Part model, mm, in its own coordinate system. Face numbers are marked on the shaded views. A direction names the side the tool comes from. Give positions to 0.01 mm unless a question says otherwise; leave off trailing zeros. Loops run counter-clockwise (first coordinate to the right, second up) from the corner with the lowest first, then second, coordinate; pieces in that order, holes last. Notation, with made-up numbers: M 33.5,-31 L 75.5,-31 A28 cw 75.5,-13 Z; hole C 43.5,27.5 d8. An arc over 180 degrees is marked long. Answer in a Markdown table with one row per item.
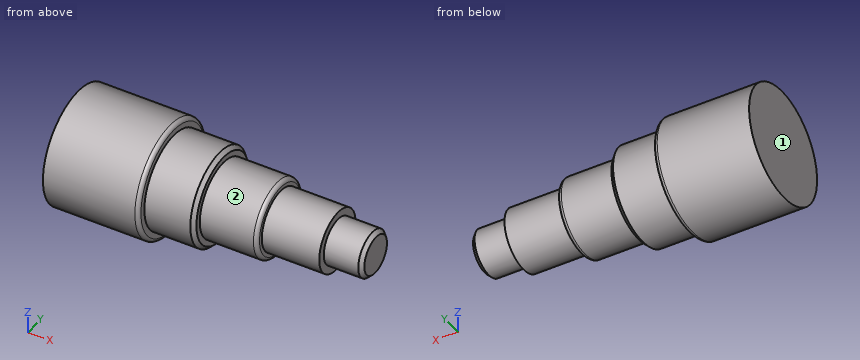
from build123d import *

# Parameters (mm, degrees)
F0_R     = 15
F1_DEPTH = 25
F2_R     = 12.5
F3_DEPTH = 13
F4_R     = 10
F5_DEPTH = 15
F6_R     = 8
F7_DEPTH = 15
F8_R     = 6
F9_DEPTH = 10
F10_R    = 1
F11_SIZE = 1


with BuildPart() as f1:
    # F0 (on Right) → F1 (new body)
    with BuildSketch(Plane.YZ):
        Circle(F0_R)
    extrude(amount=-F1_DEPTH)

    # F2 (on face) → F3 (join)
    with BuildSketch(Plane.YZ):
        Circle(F2_R)
    extrude(amount=F3_DEPTH)

    # F4 (on face) → F5 (join)
    with BuildSketch(Plane.YZ.offset(13)):
        Circle(F4_R)
    extrude(amount=F5_DEPTH)

    # F6 (on face) → F7 (join)
    with BuildSketch(Plane.YZ.offset(28)):
        Circle(F6_R)
    extrude(amount=F7_DEPTH)

    # F8 (on face) → F9 (join)
    with BuildSketch(Plane.YZ.offset(43)):
        Circle(F8_R)
    extrude(amount=F9_DEPTH)

    # F10
    f10_edges = [f1.edges().sort_by_distance(p)[0] for p in [
        (0, -15, 0),
        (28, -10, 0),
    ]]
    fillet(f10_edges, radius=F10_R)

    # F11
    f11_edges = [f1.edges().sort_by_distance(p)[0] for p in [
        (13, -12.5, 0),
        (53, -6, 0),
    ]]
    chamfer(f11_edges, length=F11_SIZE)


solid = f1.part
(1) Saw through at A-A (y = 0). Write the cut outline in (x, z), plus the area to 3 significant figures.
Recorded:
| item | result |
|---|---|
| outline | M -25,-15 L -1,-15 A1 ccw 0,-14 L 0,-12.5 L 12,-12.5 L 13,-11.5 L 13,-10 L 27,-10 A1 ccw 28,-9 L 28,-8 L 43,-8 L 43,-6 L 52,-6 L 53,-5 L 53,5 L 52,6 L 43,6 L 43,8 L 28,8 L 28,9 A1 ccw 27,10 L 13,10 L 13,11.5 L 12,12.5 L 0,12.5 L 0,14 A1 ccw -1,15 L -25,15 Z |
| area | 1,730 mm^2 |
(2) Saw through at B-B (x = -14.5). Write the cut outline in (y, z).
Recorded:
| item | result |
|---|---|
| outline | C 0,0 d30 |
(3) Saw through at C-C (x = 44). Write the cut outline in (y, z), plus the area to 3 significant figures.
Recorded:
| item | result |
|---|---|
| outline | C 0,0 d12 |
| area | 113 mm^2 |
(4) Which spindle directions (+Z, -Z, +X, -X, +Y, -Y) get a long thin tool onto all of the face, cutting with end or side? Do the marked faces 1 and 2. Say none if no direction does.
Recorded:
| item | result |
|---|---|
| face 1 | +Z, -Z, -X, +Y, -Y |
| face 2 | +X |
(5) Pin check, flat tips, straight feed: pin 1 Ø1 at (x, y) = (-10.5, 2.5) entering from +Z; pin 2 Ø8 at (x, y) = (27.5, -1.5) entering from +Z; pin 3 Ø8 at (x, z) = (-16, 11.5) entering from +Y. Stop position of each tip, or through.
Recorded:
| item | result |
|---|---|
| pin 1 | stops at z = 14.87 |
| pin 2 | stops at z = 10 |
| pin 3 | stops at y = 12.99 |
(6) Drill centre lines: line 1 along X through (y, z) = (3.25, -10.5); line 2 along X through (y, z) = (-5.5, -7.25); line 3 along Z through (x, y) = (-19, -0.5). Where is each one in solid material? Low to high.
Recorded:
| item | result |
|---|---|
| line 1 | x = -25 to 13 |
| line 2 | x = -25 to 27.99 |
| line 3 | z = -14.99 to 14.99 |
